```python
from build123d import *

# Parameters (mm, degrees)
F0_W     = 72
F0_H     = 120
F0_W_2   = 52
F0_H_2   = 85
F1_DEPTH = 15
F2_DEPTH = 14


with BuildPart() as f1:
    # F0 (on Top) → F1 (new body)
    with BuildSketch(Plane.XY):
        Rectangle(F0_W, F0_H)
        with Locations((0, 7.5)):
            Rectangle(F0_W_2, F0_H_2, mode=Mode.SUBTRACT)
    extrude(amount=F1_DEPTH)

    # F0 (on Top) → F2 (join)
    with BuildSketch(Plane.XY):
        with Locations((0, 7.5)):
            Rectangle(F0_W_2, F0_H_2)
    extrude(amount=F2_DEPTH)


solid = f1.part
```
Work out the finished part from the listing and answer in its coordinate system (mm). Round coordinates to 2 decimals unless told otherwise and drop trailing zeros. Write each loop counter-clockwise with the first axis right and the second up, starting at its lowest first coordinate (ties: lowest second). Pieces come first, ordered by that corner, then holes.
1) Determine the mould class of faces 1 (the face through (-1, 60, 7)), 2 (the face through (0, 8, 14)), 3 (the face through (-1, 1, 0)) for opening direction Z: pulls with the +Z half, pulls with the -Z half, needs draft (parallel to the pull), parting line crosses it, or undercut.
2) Consider probe 1 along Z at (x, y) = (-9.5, 21.5). Determine where the line is inside the solid, lowest interval first.
3) A flat-ended cylindrical pin translates along its axis: P1, Ø10, axis at x = -6, y = 42, coming from the +Z side. Find the tip coordinate at first contact, or state that the pin passes through.
4) A cutting plane is placed at B-B on x = 8. Determine the outline of the cut face in (y, z).
5) A cutting plane is placed at A-A on y = -20. Determine the outline of the cut face in (x, z), and give its area (3 significant figures).
Entries:
1. face 1: needs draft
1. face 2: pulls with the +Z half
1. face 3: pulls with the -Z half
2. probe 1: z = 0 to 14
3. P1: stops at z = 14
4. outline: (-60, 0) - (60, 0) - (60, 15) - (50, 15) - (50, 14) - (-35, 14) - (-35, 15) - (-60, 15) - close
5. outline: (-36, 0) - (36, 0) - (36, 15) - (26, 15) - (26, 14) - (-26, 14) - (-26, 15) - (-36, 15) - close
5. area: 1,030 mm2
